Geometry check sheet. Reference: the model listing, model coordinates, mm. A direction names the side the tool comes from. Coordinates: 2 decimals unless noted, no trailing zeros. Order: outer loops, then holes, each group sorted by start corner. A loop starts at its lowest first (then second) coordinate and runs counter-clockwise, first axis right, second up. Notation, with made-up numbers: M 0,53.25 L 36,53.25 A32 cw 36,85.25 Z; hole C 67,14.25 d3. An arc over 180 degrees is marked long. One line per item, written item: value. Start each with the question number.
1) Sectioned sample at A-A, the plane y = 0. Enter the section's corners in (x, z) (3 decimals).
2) Sectioned sample at C-C, the plane y = 37.5. Enter the section's corners in (x, z).
3) Access from +Z, -Z, +X, -X, +Y, -Y to the whole of each face (thin tool, end or side, straight path). Record for faces 4 (the cylindrical face through (46.33, -29.55, 5.07)), 5 (the flat face through (-17, 42, 6)).
4) Draft check along Y on faces 1 (the flat face through (-42, 17, 6)), 2 (the flat face through (39, -44, 10)), 3 (the cylindrical face through (-46.23, -35.44, 10.99)). Enter one of: pulls with the +Y half, pulls with the -Y half, needs draft (parallel to the pull), parting line crosses it, or undercut.
5) Thickness scan on L1, parallel to Y at x = 0, z = 8.75 (3 decimals); L2, parallel to Y at x = 45, z = 8.5; L3, parallel to X at y = -19.5, z = 7.75. Record the ranges inside material, lowest first. Write a range as from..to.
6) Sectioned sample at D-D, the plane x = 27. Enter the section's corners in (y, z).
7) Go/stop test with flat-tipped pins: P1, Ø2, axis at x = -11, z = 10, coming from the +Y side; P2, Ø3, axis at x = -23, z = 5.5, coming from the +Y side; P3, Ø1.2, axis at x = 17.5, y = -42, coming from the +Z side. Record where each tip stops, or that it passes through.
```python
from build123d import *

# Parameters (mm, degrees)
SKETCH1_R           = 59.5
BOSS_EXTRUDE1_DEPTH = 10
SKETCH4_R           = 23.525
CUT_EXTRUDE2_DEPTH  = 7
SKETCH5_R           = 18
CUT_EXTRUDE3_DEPTH  = 85.436366573
SKETCH7_R           = 2
CUT_EXTRUDE4_DEPTH  = 4
SKETCH8_R           = 1.5
CUT_EXTRUDE5_DEPTH  = 85.737830985
SKETCH10_R          = 58.25
SKETCH10_R_2        = 57.25
SKETCH10_R_3        = 56.25
BOSS_EXTRUDE2_DEPTH = 2


with BuildPart() as part:
    # Sketch1 → Boss-Extrude1 (new body)
    with BuildSketch(Plane.XY):
        Circle(SKETCH1_R)
    extrude(amount=BOSS_EXTRUDE1_DEPTH)

    # Sketch4 → Cut-Extrude2 (cut)
    with BuildSketch(Plane.XY.offset(10)):
        Circle(SKETCH4_R)
    extrude(amount=-CUT_EXTRUDE2_DEPTH, mode=Mode.SUBTRACT)

    # Sketch5 → Cut-Extrude3 (cut, through all)
    with BuildSketch(Plane.XY.offset(3)):
        Circle(SKETCH5_R)
    extrude(amount=-CUT_EXTRUDE3_DEPTH, mode=Mode.SUBTRACT)

    # Sketch7 → Cut-Extrude4 (cut)
    with BuildSketch(Plane.XY.offset(10)):
        with Locations((45, 0)):
            Circle(SKETCH7_R)
        with Locations((41.574578963, -17.220754456)):
            Circle(SKETCH7_R)
        with Locations((31.819805153, -31.819805153)):
            Circle(SKETCH7_R)
        with Locations((17.220754456, -41.574578963)):
            Circle(SKETCH7_R)
        with Locations((0, -45)):
            Circle(SKETCH7_R)
        with Locations((-17.220754456, -41.574578963)):
            Circle(SKETCH7_R)
        with Locations((-31.819805153, -31.819805153)):
            Circle(SKETCH7_R)
        with Locations((-41.574578963, -17.220754456)):
            Circle(SKETCH7_R)
        with Locations((-45, 0)):
            Circle(SKETCH7_R)
        with Locations((-41.574578963, 17.220754456)):
            Circle(SKETCH7_R)
        with Locations((-31.819805153, 31.819805153)):
            Circle(SKETCH7_R)
        with Locations((-17.220754456, 41.574578963)):
            Circle(SKETCH7_R)
        with Locations((0, 45)):
            Circle(SKETCH7_R)
        with Locations((17.220754456, 41.574578963)):
            Circle(SKETCH7_R)
        with Locations((31.819805153, 31.819805153)):
            Circle(SKETCH7_R)
        with Locations((41.574578963, 17.220754456)):
            Circle(SKETCH7_R)
    extrude(amount=-CUT_EXTRUDE4_DEPTH, mode=Mode.SUBTRACT)

    # Sketch8 → Cut-Extrude5 (cut, through all)
    with BuildSketch(Plane.XY.offset(10)):
        with Locations((30.000792583, 44.899359064)):
            Circle(SKETCH8_R)
        with Locations((52.962405142, 10.534877389)):
            Circle(SKETCH8_R)
        with Locations((44.899359064, -30.000792583)):
            Circle(SKETCH8_R)
        with Locations((10.534877389, -52.962405142)):
            Circle(SKETCH8_R)
        with Locations((-30.000792583, -44.899359064)):
            Circle(SKETCH8_R)
        with Locations((-52.962405142, -10.534877389)):
            Circle(SKETCH8_R)
        with Locations((-44.899359064, 30.000792583)):
            Circle(SKETCH8_R)
        with Locations((-10.534877389, 52.962405142)):
            Circle(SKETCH8_R)
    extrude(amount=-CUT_EXTRUDE5_DEPTH, mode=Mode.SUBTRACT)

    # Sketch10 → Boss-Extrude2 (add)
    # profile 1 of 2: a face of its own
    with BuildSketch(Plane.XY.offset(10)):
        Circle(SKETCH10_R)
        Circle(SKETCH10_R_2, mode=Mode.SUBTRACT)
    # profile 2 of 2: a face of its own
    with BuildSketch(Plane.XY.offset(10)):
        Circle(SKETCH10_R_2)
        Circle(SKETCH10_R_3, mode=Mode.SUBTRACT)
    extrude(amount=BOSS_EXTRUDE2_DEPTH)


solid = part.part
```
Final values:
1. outline: M -59.5,0 L -18,0 L -18,3 L -23.525,3 L -23.525,10 L -43,10 L -43,6 L -47,6 L -47,10 L -56.25,10 L -56.25,12 L -58.25,12 L -58.25,10 L -59.5,10 Z; M 18,0 L 59.5,0 L 59.5,10 L 58.25,10 L 58.25,12 L 56.25,12 L 56.25,10 L 47,10 L 47,6 L 43,6 L 43,10 L 23.525,10 L 23.525,3 L 18,3 Z
2. outline: M -46.2,0 L 46.2,0 L 46.2,10 L 44.57,10 L 44.57,12 L 41.93,12 L 41.93,10 L -41.93,10 L -41.93,12 L -44.57,12 L -44.57,10 L -46.2,10 Z
3. face 4: +Z, -Z
3. face 5: +Z
4. face 1: undercut
4. face 2: needs draft
4. face 3: parting line crosses it
5. L1: y = -59.5..-47, -43..-23.525, 23.525..43, 47..59.5
5. L2: y = -38.93..-31.5, -28.5..-2, 2..38.93
5. L3: x = -56.21..-13.16, 13.16..56.21
6. outline: M -53.02,0 L 53.02,0 L 53.02,10 L 51.61,10 L 51.61,12 L 49.35,12 L 49.35,10 L -49.35,10 L -49.35,12 L -51.61,12 L -51.61,10 L -53.02,10 Z
7. P1: stops at y = 58.65
7. P2: stops at y = 55.48
7. P3: stops at z = 6
